The listing builds one solid part. Answer for the finished solid, in the listing's coordinates (mm). Face numbers are marked on the shaded views. A direction names the side the tool comes from. Give positions to 0.01 mm unless a question says otherwise; leave off trailing zeros. Loops run counter-clockwise (first coordinate to the right, second up) from the corner with the lowest first, then second, coordinate; pieces in that order, holes last. Notation, with made-up numbers: M 42.5,-14 L 78.5,-14 A24 ccw 78.5,16 Z; hole C 42,52.5 d9. An arc over 180 degrees is marked long. Use one line per item in the form item = value. Start each with the question number.
1. Straight lines are drawn through the part: line 1 (Z direction, x = 3.5, y = -74.5); line 2 (Z direction, x = -10, y = 41.5); line 3 (Z direction, x = -1.5, y = 37). For each, find the intervals that lie inside material, in ascending order. Write a range as from..to.
2. For the marked faces 1, 2, 3 and 4, determine the directions among +Z, -Z, +X, -X, +Y, -Y from which every point of the face is accessible in a straight line to the end or side of a thin tool.
3. The part is cut by section A-A (y = -49.5). Write down the section's boundary in (x, z).
4. Each of these flat-tipped pins is pushed along its axis until it touches: pin 1 Ø10 at (x, z) = (-18.5, -23.5) entering from -Y; pin 2 Ø3 at (x, y) = (11, 26.5) entering from +Z; pin 3 Ø17.5 at (x, z) = (13.5, -5) entering from -Y. Where does it stop, or does it pass through?
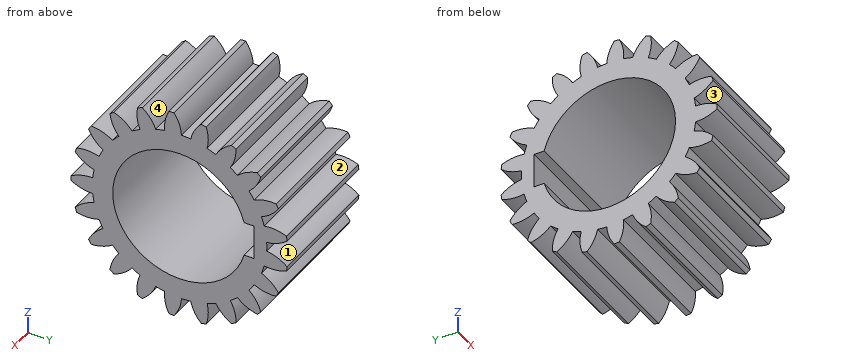
from build123d import *

# Parameters (mm, degrees)
BOSS_EXTRU_1_DEPTH = 77


with BuildPart() as part:
    # Esquisse1 → Boss.-Extru.1 (new body)
    with BuildSketch(Plane(origin=(40.821362871, 0, 0), x_dir=(0, 0, -1), z_dir=(1, 0, 0))):
        with BuildLine():
            ThreePointArc((-67.612453277, -3.518534748), (-61.812081339, -7.771811815), (-55.046417386, -10.213219545))
            ThreePointArc((-55.046417386, -10.213219545), (-55.34381354, -13.139028919), (-55.485808315, -16.076484017))
            ThreePointArc((-55.485808315, -16.076484017), (-62.539778332, -17.482253352), (-68.909282961, -20.82352425))
            ThreePointArc((-68.909282961, -20.82352425), (-68.807062006, -22.442850841), (-68.666793133, -24.059326134))
            ThreePointArc((-68.666793133, -24.059326134), (-61.870440021, -26.413952393), (-54.685737973, -26.752680769))
            ThreePointArc((-54.685737973, -26.752680769), (-54.107524198, -29.636163697), (-53.377380454, -32.484969601))
            ThreePointArc((-53.377380454, -32.484969601), (-59.70360459, -35.907478712), (-64.805273114, -40.977750767))
            ThreePointArc((-64.805273114, -40.977750767), (-64.230288656, -42.495005065), (-63.619787079, -43.99831992))
            ThreePointArc((-63.619787079, -43.99831992), (-56.431338594, -44.245076494), (-49.465990757, -42.451028013))
            ThreePointArc((-49.465990757, -42.451028013), (-48.063543885, -45.035974383), (-46.526138097, -47.543002188))
            ThreePointArc((-46.526138097, -47.543002188), (-51.562503575, -52.67814612), (-54.943030357, -59.026903409))
            ThreePointArc((-54.943030357, -59.026903409), (-53.94637229, -60.307270712), (-52.919883753, -61.563849007))
            ThreePointArc((-52.919883753, -61.563849007), (-45.978065087, -59.680810492), (-39.850973185, -55.913394235))
            ThreePointArc((-39.850973185, -55.913394235), (-37.748906774, -57.970120218), (-35.540844194, -59.9126095))
            ThreePointArc((-35.540844194, -59.9126095), (-38.839847839, -66.30410818), (-40.198858239, -73.367235757))
            ThreePointArc((-40.198858239, -73.367235757), (-38.869084006, -74.296949811), (-37.51781652, -75.195139051))
            ThreePointArc((-37.51781652, -75.195139051), (-31.439438727, -71.349621682), (-26.695021762, -65.943589116))
            ThreePointArc((-26.695021762, -65.943589116), (-24.080113637, -67.289345583), (-21.397590315, -68.494697646))
            ThreePointArc((-21.397590315, -68.494697646), (-22.666101177, -75.574638368), (-21.882841157, -82.724546352))
            ThreePointArc((-21.882841157, -82.724546352), (-20.338107034, -83.220997983), (-18.782126645, -83.680990111))
            ThreePointArc((-18.782126645, -83.680990111), (-14.107280265, -78.214684982), (-11.167100506, -71.650385825))
            ThreePointArc((-11.167100506, -71.650385825), (-8.271696731, -72.165596408), (-5.353066636, -72.526710431))
            ThreePointArc((-5.353066636, -72.526710431), (-4.478371957, -79.666009392), (-1.622437607, -86.267397081))
            ThreePointArc((-1.622437607, -86.267397081), (0, -86.286474383), (1.622437607, -86.267397081))
            ThreePointArc((1.622437607, -86.267397081), (4.478371957, -79.666009392), (5.353066636, -72.526710431))
            ThreePointArc((5.353066636, -72.526710431), (8.271696731, -72.165596408), (11.167100506, -71.650385825))
            ThreePointArc((11.167100506, -71.650385825), (14.107280265, -78.214684982), (18.782126645, -83.680990111))
            ThreePointArc((18.782126645, -83.680990111), (20.338107034, -83.220997983), (21.882841157, -82.724546352))
            ThreePointArc((21.882841157, -82.724546352), (22.666101177, -75.574638368), (21.397590315, -68.494697646))
            ThreePointArc((21.397590315, -68.494697646), (24.080113637, -67.289345583), (26.695021762, -65.943589116))
            ThreePointArc((26.695021762, -65.943589116), (31.439438727, -71.349621682), (37.51781652, -75.195139051))
            ThreePointArc((37.51781652, -75.195139051), (38.869084006, -74.296949811), (40.198858239, -73.367235757))
            ThreePointArc((40.198858239, -73.367235757), (38.839847839, -66.30410818), (35.540844194, -59.9126095))
            ThreePointArc((35.540844194, -59.9126095), (37.748906774, -57.970120218), (39.850973185, -55.913394235))
            ThreePointArc((39.850973185, -55.913394235), (45.978065087, -59.680810492), (52.919883753, -61.563849007))
            ThreePointArc((52.919883753, -61.563849007), (53.94637229, -60.307270712), (54.943030357, -59.026903409))
            ThreePointArc((54.943030357, -59.026903409), (51.562503575, -52.67814612), (46.526138097, -47.543002188))
            ThreePointArc((46.526138097, -47.543002188), (48.063543885, -45.035974383), (49.465990757, -42.451028013))
            ThreePointArc((49.465990757, -42.451028013), (56.431338594, -44.245076494), (63.619787079, -43.99831992))
            ThreePointArc((63.619787079, -43.99831992), (64.230288656, -42.495005065), (64.805273114, -40.977750767))
            ThreePointArc((64.805273114, -40.977750767), (59.70360459, -35.907478712), (53.377380454, -32.484969601))
            ThreePointArc((53.377380454, -32.484969601), (54.107524198, -29.636163697), (54.685737973, -26.752680769))
            ThreePointArc((54.685737973, -26.752680769), (61.870440021, -26.413952393), (68.666793133, -24.059326134))
            ThreePointArc((68.666793133, -24.059326134), (68.807062006, -22.442850841), (68.909282961, -20.82352425))
            ThreePointArc((68.909282961, -20.82352425), (62.539778332, -17.482253352), (55.485808315, -16.076484017))
            ThreePointArc((55.485808315, -16.076484017), (55.34381354, -13.139028919), (55.046417386, -10.213219545))
            ThreePointArc((55.046417386, -10.213219545), (61.812081339, -7.771811815), (67.612453277, -3.518534748))
            ThreePointArc((67.612453277, -3.518534748), (67.270025941, -1.93252994), (66.890400614, -0.355015331))
            ThreePointArc((66.890400614, -0.355015331), (59.819018318, 0.960367828), (52.664078611, 0.224488613))
            ThreePointArc((52.664078611, 0.224488613), (51.662562176, 2.989587128), (50.515981046, 5.697751946))
            ThreePointArc((50.515981046, 5.697751946), (56.261447972, 10.024909239), (60.550450236, 15.798914782))
            ThreePointArc((60.550450236, 15.798914782), (59.755752861, 17.213525617), (58.928012629, 18.609059149))
            ThreePointArc((58.928012629, 18.609059149), (51.783076015, 17.781677003), (45.16291441, 14.969535335))
            ThreePointArc((45.16291441, 14.969535335), (43.390865445, 17.31658613), (41.496978105, 19.566474063))
            ThreePointArc((41.496978105, 19.566474063), (45.711738053, 25.394894004), (48.10827397, 32.176582292))
            ThreePointArc((48.10827397, 32.176582292), (46.931918906, 33.294104773), (45.729612121, 34.383657949))
            ThreePointArc((45.729612121, 34.383657949), (39.145980162, 31.487027033), (33.64882707, 26.848494041))
            ThreePointArc((33.64882707, 26.848494041), (31.263699902, 28.568951352), (28.790786553, 30.160649984))
            ThreePointArc((28.790786553, 30.160649984), (31.100339606, 36.972451884), (31.391466441, 44.159240151))
            ThreePointArc((31.391466441, 44.159240151), (29.937977999, 44.880377502), (28.467934894, 45.567138742))
            ThreePointArc((28.467934894, 45.567138742), (23.030592182, 40.858637423), (19.14489378, 34.805867119))
            ThreePointArc((19.14489378, 34.805867119), (16.358617425, 35.746860765), (13.526407269, 36.538940686))
            ThreePointArc((13.526407269, 36.538940686), (13.725539503, 43.728866053), (11.885389361, 50.682176624))
            ThreePointArc((11.885389361, 50.682176624), (10.283916366, 50.942852626), (8.676756723, 51.165800179))
            ThreePointArc((8.676756723, 51.165800179), (4.868835019, 45.063799464), (2.93985266, 38.134607051))
            ThreePointArc((2.93985266, 38.134607051), (0, 38.212525617), (-2.93985266, 38.134607051))
            ThreePointArc((-2.93985266, 38.134607051), (-4.868835019, 45.063799464), (-8.676756723, 51.165800179))
            ThreePointArc((-8.676756723, 51.165800179), (-10.283916366, 50.942852626), (-11.885389361, 50.682176624))
            ThreePointArc((-11.885389361, 50.682176624), (-13.725539503, 43.728866053), (-13.526407269, 36.538940686))
            ThreePointArc((-13.526407269, 36.538940686), (-16.358617425, 35.746860765), (-19.14489378, 34.805867119))
            ThreePointArc((-19.14489378, 34.805867119), (-23.030592182, 40.858637423), (-28.467934894, 45.567138742))
            ThreePointArc((-28.467934894, 45.567138742), (-29.937977999, 44.880377502), (-31.391466441, 44.159240151))
            ThreePointArc((-31.391466441, 44.159240151), (-31.100339606, 36.972451884), (-28.790786553, 30.160649984))
            ThreePointArc((-28.790786553, 30.160649984), (-31.263699902, 28.568951352), (-33.64882707, 26.848494041))
            ThreePointArc((-33.64882707, 26.848494041), (-39.145980162, 31.487027033), (-45.729612121, 34.383657949))
            ThreePointArc((-45.729612121, 34.383657949), (-46.931918906, 33.294104773), (-48.10827397, 32.176582292))
            ThreePointArc((-48.10827397, 32.176582292), (-45.711738053, 25.394894004), (-41.496978105, 19.566474063))
            ThreePointArc((-41.496978105, 19.566474063), (-43.390865445, 17.31658613), (-45.16291441, 14.969535335))
            ThreePointArc((-45.16291441, 14.969535335), (-51.783076015, 17.781677003), (-58.928012629, 18.609059149))
            ThreePointArc((-58.928012629, 18.609059149), (-59.755752861, 17.213525617), (-60.550450236, 15.798914782))
            ThreePointArc((-60.550450236, 15.798914782), (-56.261447972, 10.024909239), (-50.515981046, 5.697751946))
            ThreePointArc((-50.515981046, 5.697751946), (-51.662562176, 2.989587128), (-52.664078611, 0.224488613))
            ThreePointArc((-52.664078611, 0.224488613), (-59.819018318, 0.960367828), (-66.890400614, -0.355015331))
            ThreePointArc((-66.890400614, -0.355015331), (-67.270025941, -1.93252994), (-67.612453277, -3.518534748))
        make_face()
        with BuildLine():
            Line((-11, 30.213525617), (11, 30.213525617))
            Line((11, 30.213525617), (11, 23.765322167))
            ThreePointArc((11, 23.765322167), (0, -59.786474383), (-11, 23.765322167))
            Line((-11, 23.765322167), (-11, 30.213525617))
        make_face(mode=Mode.SUBTRACT)
    extrude(amount=-BOSS_EXTRU_1_DEPTH)


solid = part.part
Derived:
q1.line_1 = -38.57..-36.09, -22.61..-12.17, -5.32..5.32, 12.17..22.61, 36.09..38.57
q1.line_2 = -31.52..-23.61, -13.88..-3.61, 3.61..13.88, 23.61..31.52
q1.line_3 = -31.11..-20.28, -13.6..13.6, 20.28..31.11
q2.face_1 = +X, -X, +Y
q2.face_2 = +X, -X
q2.face_3 = +X, -X, -Y
q2.face_4 = +Z, +X, -X
q3.outline = M -36.18,-48.8 L 40.82,-48.8 L 40.82,-27.72 L -36.18,-27.72 Z; M -36.18,27.72 L 40.82,27.72 L 40.82,48.8 L -36.18,48.8 Z
q4.pin_1 = -83.68
q4.pin_2 = 46.89
q4.pin_3 = -86.29
